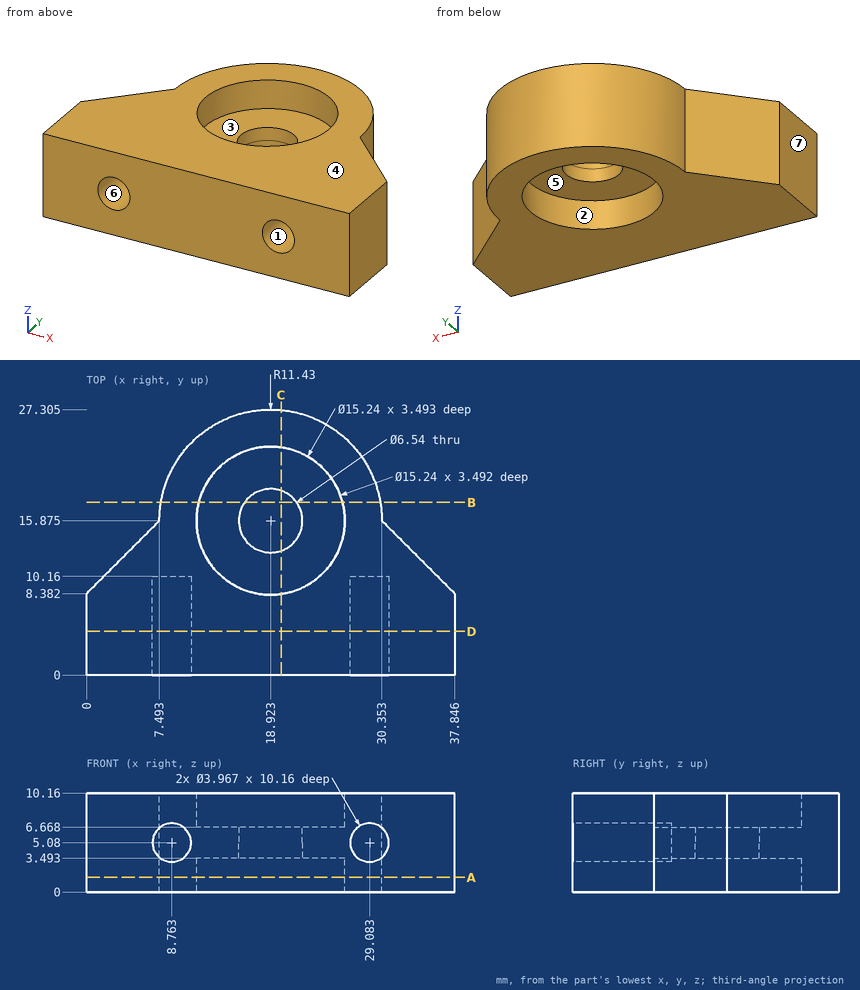
Job drawing, mm, ordinate dimensions from the low corner. One solid piece. A direction names the side the tool comes from. Coordinates: 2 decimals unless noted, no trailing zeros. Loops run counter-clockwise (first coordinate to the right, second up) from the corner with the lowest first, then second, coordinate; pieces in that order, holes last. Notation, with made-up numbers: (-17, 56.5) - (27, 56.5) arc R19 cw to (27, 90.5) - close; hole circle Ø5 at (89.5, 12.5). An arc over 180 degrees is marked (long way). Write item = value, one per line. Start each with the question number.
Q1. Which spindle directions (+Z, -Z, +X, -X, +Y, -Y) get a long thin tool onto all of the face, cutting with end or side? Do the marked faces 1, 2 and 3. Say none if no direction does.
Q2. Cut at A-A, the plane z = 1.5. List the corners of the cut face in (x, y) (1 decimal).
Q3. Pull direction X, two halves, no side cores. Call the marked faces 4, 5, 6 and 7: pulls with the +X half, pulls with the -X half, needs draft (parallel to the pull), parting line crosses it, or undercut.
Q4. Cut at B-B, the plane y = 17.75. List the corners of the cut face in (x, z).
Q5. Drill centre lines: L1, parallel to X at y = 4.25, z = 5.08 (1 decimal); L2, parallel to X at y = 9.5, z = 6 (1 decimal); L3, parallel to Z at x = 13.5, y = 11.5. Where is each one in solid material? Low to high.
Q6. Flat gauge pins, fed straight in: pin 1 Ø3 at (y, z) = (13, 3) entering from +X; pin 2 Ø6 at (y, z) = (22.5, 2.5) entering from +X; pin 3 Ø2 at (x, y) = (23, 20) entering from +Z; pin 4 Ø6 at (x, y) = (18.923, 15.875) entering from -Z. Where does each tip first touch, or does it go through?
Q7. Cut at C-C, the plane x = 20. List the corners of the cut face in (y, z) (1 decimal), then the cut area to 3 significant figures.
Q8. Cut at D-D, the plane y = 4.5. List the corners of the cut face in (x, z) (1 decimal).
Computed:
q1.face_1 = -Y
q1.face_2 = -Z
q1.face_3 = +Z
q2.outline = (0, 0) - (37.8, 0) - (37.8, 8.4) - (30.4, 15.9) arc R11.4 ccw to (7.5, 15.9) - (0, 8.4) - close; hole circle Ø15.2 at (18.9, 15.9)
q3.face_4 = needs draft
q3.face_5 = undercut
q3.face_6 = undercut
q3.face_7 = pulls with the -X half
q4.outline = (7.65, 0) - (11.54, 0) - (11.54, 3.49) - (16.24, 3.49) - (16.24, 6.67) - (11.54, 6.67) - (11.54, 10.16) - (7.65, 10.16) - close; (21.6, 3.49) - (26.31, 3.49) - (26.31, 0) - (30.2, 0) - (30.2, 10.16) - (26.31, 10.16) - (26.31, 6.67) - (21.6, 6.67) - close
q5.L1 = 0 to 6.8, 10.7 to 27.1, 31.1 to 37.8
q5.L2 = 1.1 to 7, 10.5 to 27.3, 30.8 to 36.7
q5.L3 = 3.49 to 6.67
q6.pin_1 = 34.73
q6.pin_2 = 29.76
q6.pin_3 = 6.67
q6.pin_4 = through
q7.outline = (0, 0) - (8.3, 0) - (8.3, 3.5) - (12.8, 3.5) - (12.8, 6.7) - (8.3, 6.7) - (8.3, 10.2) - (0, 10.2) - close; (19, 3.5) - (23.4, 3.5) - (23.4, 0) - (27.3, 0) - (27.3, 10.2) - (23.4, 10.2) - (23.4, 6.7) - (19, 6.7) - close
q7.area = 152 mm²
q8.outline = (0, 0) - (37.8, 0) - (37.8, 10.2) - (0, 10.2) - close; hole circle Ø4 at (8.8, 5.1); hole circle Ø4 at (29.1, 5.1)
